Design review of the part built by this model. Coordinates are the model's own, in mm. Face numbers are marked on the shaded views. A direction names the side the tool comes from. Round coordinates to 2 decimals unless told otherwise and drop trailing zeros. Order: outer loops, then holes, each group sorted by start corner. A loop starts at its lowest first (then second) coordinate and runs counter-clockwise, first axis right, second up. Notation, with made-up numbers: (82, -34) - (113, -34) arc R14 ccw to (113, -7) - close; hole circle Ø11 at (69.25, 7). An arc over 180 degrees is marked (long way). Use CSV: the item, a comma, the result in double quotes.
Autodesk Fusion 360 part; units mm, degrees
sketch "Sketch1" plane through (0, 0, 0) normal (0, 0, 1) x (1, 0, 0)
  line L0 (0, 0) -> (-35, 0)
  line L1 (-35, 0) -> (-35, 16)
  line L2 (-35, 16) -> (0, 16)
  line L3 (0, 16) -> (0, 0)
  dimension "d14" = 16
  dimension "d15" = 35
extrude "Extrude1" add sketch "Sketch1" along normal blind 3.5
sketch "Sketch3" plane through (0, 0, 0) normal (0, 1, 0) x (1, 0, 0)
  line L0 (0, -3.5) -> (-6, -3.5)
  line L1 (-6, -3.5) -> (-6, -15.5)
  line L2 (-6, -15.5) -> (0, -15.5)
  line L3 (0, -15.5) -> (0, -3.5)
  line L4 (-35, -3.5) -> (-29, -3.5)
  line L5 (-29, -3.5) -> (-29, -15.5)
  line L6 (-29, -15.5) -> (-35, -15.5)
  line L7 (-35, -15.5) -> (-35, -3.5)
  point P0 (0, -3.5)
  point P1 (-35, -3.5)
  dimension "d17" = 12
  dimension "d19" = 23
extrude "Extrude3" add sketch "Sketch3" along normal blind 3
sketch "Sketch4" plane through (0, 0, 3.5) normal (0, 0, 1) x (-1, 0, 0)
  line L0 (6, 0) -> (6, -3)
  line L1 (6, -3) -> (0, -3)
  line L2 (0, -3) -> (0, -16)
  line L3 (0, -16) -> (35, -16)
  line L4 (35, -16) -> (35, -3)
  line L5 (35, -3) -> (29, -3)
  line L6 (29, -3) -> (29, 0)
  line L7 (29, 0) -> (6, 0)
  line L8 (0, -16) -> (35, 0) construction
  line L9 (35, -16) -> (0, 0) construction
  circle A0 centre (17.5, -8) radius 3.75
  dimension "d22" = 7.5
extrude "Extrude4" cut sketch "Sketch4" against normal up to surface (3.5 mm away) contours A0
sketch "Sketch7" plane through (0, 3, 0) normal (0, 1, 0) x (-1, 0, 0)
  line L0 (0, 15.5) -> (0, 3.5)
  line L1 (0, 3.5) -> (6, 3.5)
  line L2 (6, 3.5) -> (6, 15.5)
  line L3 (6, 15.5) -> (0, 15.5)
  line L4 (0, 9.5) -> (35, 9.5) construction
  line L5 (35, 3.5) -> (35, 15.5) construction
  circle A0 centre (3.5, 9.5) radius 0.9
  circle A1 centre (31.5, 9.5) radius 0.9
  line L6 (32.4, 9.5) -> (32.3186, 9.874) construction
  point P0 (17.5, 9.5)
  dimension "d30" = 1.8
  dimension "d31" = 14
  dimension "d32" = 1.8
  dimension "d33" = 14
extrude "Extrude6" cut sketch "Sketch7" against normal up to surface (3 mm away) contours A0 | A1
fillet "Fillet1" radius 1.5 2 edges at (-3, 3, 3.5) (-32, 3, 3.5)
fillet "Fillet2" radius 1.5 2 edges at (0, 16, 1.75) (-35, 16, 1.75)
extrude "Extrude2" [suppressed]
hole "Hole1" [suppressed]
hole "Hole2" [suppressed]
hole "Hole3" [suppressed]
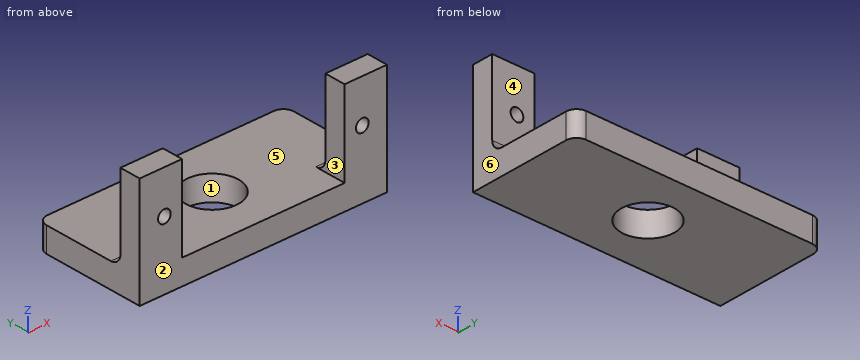
1) To check wall thickness, follow L1, parallel to Z at x = -31.5, y = 0.8; L2, parallel to X at y = 8, z = 1.05; L3, parallel to Y at x = -17.5, z = 1.9. State the ranges of each line that lie inside material, in increasing order. Write a range as from..to.
Data:
L1,"z = 0..8.6, 10.4..15.5"
L2,"x = -35..-21.25, -13.75..0"
L3,"y = 0..4.25, 11.75..16"
2) For the marked faces 5 and 6, list the 3-axis set-ups (+Z, -Z, +X, -X, +Y, -Y) from which the entire face can be reached by the end or side of a thin tool; tool diameter is ignored.
Data:
face 5,"+Z, +Y"
face 6,"+Z, -Z, +X, +Y, -Y"
3) We need section C-C (y = 8). Give the boundary of the cut face in (x, z), then the cut area to 4 significant figures.
Data:
outline,"(-35, 0) - (-21.25, 0) - (-21.25, 3.5) - (-35, 3.5) - close; (-13.75, 0) - (0, 0) - (0, 3.5) - (-13.75, 3.5) - close"
area,"96.25 mm2"
4) The part is to be moulded in two halves that separate along Y. For the marked faces 1, 2, 3 and 4, say which applies: +Y half, -Y half, draft (parallel to the pull), parting line (faces both ways), or undercut.
Data:
face 1,"undercut"
face 2,"-Y half"
face 3,"draft"
face 4,"+Y half"
5) We need section B-B (z = 9.5). Give the boundary of the cut face in (x, y), then the cut area to 3 significant figures.
Data:
outline,"(-35, 0) - (-32.4, 0) - (-32.4, 3) - (-35, 3) - close; (-30.6, 0) - (-29, 0) - (-29, 3) - (-30.6, 3) - close; (-6, 0) - (-4.4, 0) - (-4.4, 3) - (-6, 3) - close; (-2.6, 0) - (0, 0) - (0, 3) - (-2.6, 3) - close"
area,"25.2 mm2"
6) We need section D-D (x = -31.5). Give the boundary of the cut face in (y, z), then the cut area to 3 significant figures.
Data:
outline,"(0, 0) - (16, 0) - (16, 3.5) - (4.5, 3.5) arc R1.5 cw to (3, 5) - (3, 8.6) - (0, 8.6) - close; (0, 10.4) - (3, 10.4) - (3, 15.5) - (0, 15.5) - close"
area,"87.1 mm2"
7) Insertion check: pin 1 Ø2 at (x, z) = (-31.5, 9.5) entering from +Y; pin 2 Ø8 at (x, y) = (-12, 11) entering from +Z. Each pin has a flat end and moves straight along its axis. Give the tip position at first contact, or say it passes through.
Data:
pin 1,"stops at y = 3"
pin 2,"stops at z = 3.5"
8) We need section A-A (x = -17.5). Give the boundary of the cut face in (y, z).
Data:
outline,"(0, 0) - (4.25, 0) - (4.25, 3.5) - (0, 3.5) - close; (11.75, 0) - (16, 0) - (16, 3.5) - (11.75, 3.5) - close"
